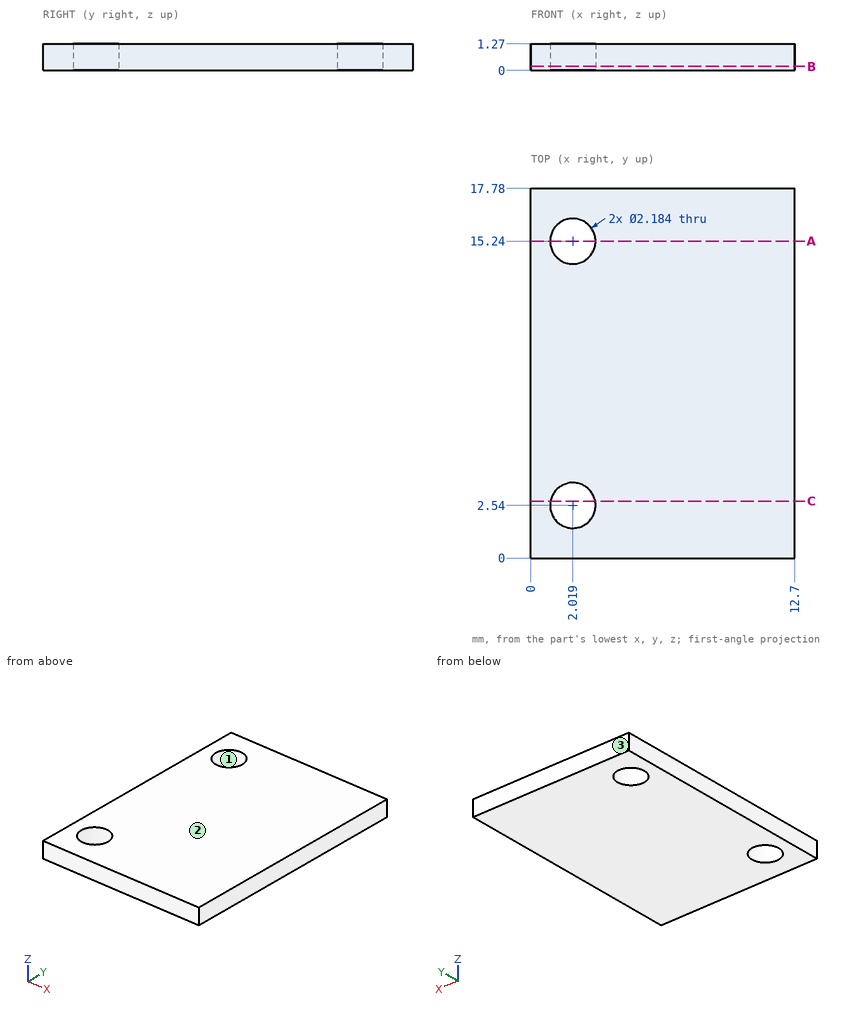
Verification items for this drawing (mm, ordinates from the low corner). Give positions to 0.01 mm unless a question says otherwise; leave off trailing zeros. Loops run counter-clockwise (first coordinate to the right, second up) from the corner with the lowest first, then second, coordinate; pieces in that order, holes last. Notation, with made-up numbers: M -5,-25 L 26,-25 A20 cw 26,0 Z; hole C -39,0.5 d6. An arc over 180 degrees is marked long. Answer as a JSON object with one key per item and string values. Group by question number.
Item 1: Sectioned sample at B-B on z = 0.2. Record the boundary of the cut face in (x, y) (1 decimal).
Item 2: Sectioned sample at C-C on y = 2.75. Record the boundary of the cut face in (x, z), plus the area to 3 significant figures.
Item 3: Material ranges on L1, parallel to Y at x = 2, z = 0.15; L2, parallel to Y at x = 3, z = 0.9 (1 decimal); L3, parallel to X at y = 15.5, z = 0.7, recorded low to high.
Item 4: Mould release check, pull along Y, two halves, no side actions. Record for the marked faces 1, 2 and 3: pulls with the +Y half, pulls with the -Y half, needs draft (parallel to the pull), parting line crosses it, or undercut.
Item 5: Sectioned sample at A-A on y = 15.24. Record the boundary of the cut face in (x, z).
Findings below:
{
 "1": {"outline": "M 0,0 L 12.7,0 L 12.7,17.8 L 0,17.8 Z; hole C 2,2.5 d2.2; hole C 2,15.2 d2.2"},
 "2": {"outline": "M 0,0 L 0.95,0 L 0.95,1.27 L 0,1.27 Z; M 3.09,0 L 12.7,0 L 12.7,1.27 L 3.09,1.27 Z", "area": "13.4 mm2"},
 "3": {"L1": "0 to 1.45, 3.63 to 14.15, 16.33 to 17.78", "L2": "0 to 2.1, 3 to 14.8, 15.7 to 17.8", "L3": "0 to 0.96, 3.08 to 12.7"},
 "4": {"face 1": "undercut", "face 2": "needs draft", "face 3": "pulls with the +Y half"},
 "5": {"outline": "M 0,0 L 0.93,0 L 0.93,1.27 L 0,1.27 Z; M 3.11,0 L 12.7,0 L 12.7,1.27 L 3.11,1.27 Z"}
}
